```python
from build123d import *

# Parameters (mm, degrees)
CROQUIS1_R              = 8.85
SALIENTE_EXTRUIR1_DEPTH = 6.45
CROQUIS2_R              = 6
SALIENTE_EXTRUIR2_DEPTH = 12.9
CROQUIS3_R              = 8.85
SALIENTE_EXTRUIR3_DEPTH = 1.4
CROQUIS4_R              = 4
CORTAR_EXTRUIR1_DEPTH   = 25.232364722
CROQUIS6_W              = 1.65
CROQUIS6_H              = 8.851
MATRIZC1_COUNT          = 2
MATRIZC1_ANGLE          = 90


with BuildPart() as part:
    # Croquis1 → Saliente-Extruir1 (new body)
    with BuildSketch(Plane(origin=(0, 0, 0), x_dir=(1, 0, 0), z_dir=(0, 1, 0))):
        with Locations(Location((0, 0, 0), (0, 0, 90))):
            Circle(CROQUIS1_R)
    extrude(amount=SALIENTE_EXTRUIR1_DEPTH)

    # Croquis2 → Saliente-Extruir2 (add)
    with BuildSketch(Plane(origin=(0, 6.45, 0), x_dir=(1, 0, 0), z_dir=(0, 1, 0))):
        with Locations(Location((0, 0, 0), (0, 0, 90))):
            Circle(CROQUIS2_R)
    extrude(amount=SALIENTE_EXTRUIR2_DEPTH)

    # Croquis3 → Saliente-Extruir3 (add)
    with BuildSketch(Plane(origin=(0, 19.35, 0), x_dir=(1, 0, 0), z_dir=(0, 1, 0))):
        with Locations(Location((0, 0, 0), (0, 0, 90))):
            Circle(CROQUIS3_R)
    extrude(amount=SALIENTE_EXTRUIR3_DEPTH)

    # Croquis4 → Cortar-Extruir1 (cut, through all)
    with BuildSketch(Plane(origin=(0, 20.75, 0), x_dir=(1, 0, 0), z_dir=(0, 1, 0))):
        with Locations(Location((0, 0, 0), (0, 0, 270))):
            Circle(CROQUIS4_R)
    extrude(amount=-CORTAR_EXTRUIR1_DEPTH, mode=Mode.SUBTRACT)

    # Croquis6 → Taladro roscado M41 (falta definir posicio) (revolve, cut)
    with BuildSketch(Plane(origin=(0, 3.225, 0), x_dir=(0, 1, 0), z_dir=(1, 0, 0))):
        with Locations((0.825, 4.4255)):
            Rectangle(CROQUIS6_W, CROQUIS6_H)
    taladro_roscado_m41_falta_definir_posic = revolve(axis=Axis((0, 3.225, -6.35), (0, 0, 1)), mode=Mode.SUBTRACT)

    # MatrizC1: Taladro roscado M41 (falta definir posicio) ×2 about axis
    matrizc1_axis = Axis((0, 6.45, 0), (0, -1, 0))
    for i in range(1, MATRIZC1_COUNT):
        add(taladro_roscado_m41_falta_definir_posic.rotate(matrizc1_axis, i * MATRIZC1_ANGLE / (MATRIZC1_COUNT - 1)), mode=Mode.SUBTRACT)


solid = part.part
```
Could you check a few things on this model? Use its own coordinates, in mm. A direction names the side the tool comes from. Coordinates: 2 decimals unless noted, no trailing zeros. Write each loop counter-clockwise with the first axis right and the second up, starting at its lowest first coordinate (ties: lowest second). Pieces come first, ordered by that corner, then holes. Notation, with made-up numbers: (49.25, -2) -> (78.25, -2) arc R23 ccw to (78.25, 28) -> close; hole circle Ø5 at (-26, 14). An arc over 180 degrees is marked (long way). Return JSON: item names as keys, results as strings.
(1) We'd pull the mould along Y, two halves only. Please class faces 4 (the cylindrical face through (-2.66, 20.04, -8.44)), 5 (the flat face through (2, 6.45, -6)), 6 (the cylindrical face through (-6.29, 4.75, 0.63)), 7 (the flat face through (2, 20.75, -4)): +Y half, -Y half, draft (parallel to the pull), parting line (faces both ways), or undercut.
Numbers:
{"face 4": "draft", "face 5": "undercut", "face 6": "undercut", "face 7": "+Y half"}
(2) Which directions (+Z, -Z, +X, -X, +Y, -Y) give clear straight access to the entire face, cutting with the end or side of a thin tool? Please do faces 1 (the flat face through (2, 19.35, -6)), 2 (the cylindrical face through (0.63, 4.75, 6.28)), 3 (the cylindrical face through (3.39, 3.18, -8.175)).
Numbers:
{"face 1": "none", "face 2": "+Z", "face 3": "+Y, -Y"}
(3) Imagine slicing it at A-A, the plane x = 0. Please give me the cut outline in (y, z) (3 decimals), then the cut area to 3 significant figures.
Numbers:
{"outline": "(0, -8.85) -> (6.45, -8.85) -> (6.45, -6) -> (19.35, -6) -> (19.35, -8.85) -> (20.75, -8.85) -> (20.75, -4) -> (0, -4) -> close; (0, 4) -> (1.575, 4) -> (1.575, 8.85) -> (0, 8.85) -> close; (4.875, 4) -> (20.75, 4) -> (20.75, 8.85) -> (19.35, 8.85) -> (19.35, 6) -> (6.45, 6) -> (6.45, 8.85) -> (4.875, 8.85) -> close", "area": "112 mm2"}
(4) Imagine slicing it at C-C, the plane z = -3. Please give me the cut outline in (x, y), then the cut area to 3 significant figures.
Numbers:
{"outline": "(-8.33, 0) -> (-2.65, 0) -> (-2.65, 20.75) -> (-8.33, 20.75) -> (-8.33, 19.35) -> (-5.2, 19.35) -> (-5.2, 6.45) -> (-8.33, 6.45) -> close; (2.65, 0) -> (8.33, 0) -> (8.33, 6.45) -> (5.2, 6.45) -> (5.2, 19.35) -> (8.33, 19.35) -> (8.33, 20.75) -> (2.65, 20.75) -> close", "area": "155 mm2"}
(5) Imagine slicing it at B-B, the plane z = 0. Please give me the cut outline in (x, y) (3 decimals).
Numbers:
{"outline": "(-8.85, 0) -> (-4, 0) -> (-4, 1.575) -> (-8.85, 1.575) -> close; (-8.85, 4.875) -> (-4, 4.875) -> (-4, 20.75) -> (-8.85, 20.75) -> (-8.85, 19.35) -> (-6, 19.35) -> (-6, 6.45) -> (-8.85, 6.45) -> close; (4, 0) -> (8.85, 0) -> (8.85, 6.45) -> (6, 6.45) -> (6, 19.35) -> (8.85, 19.35) -> (8.85, 20.75) -> (4, 20.75) -> close"}
(6) I'm going to push flat-ended pins straight in: pin 1 (3 mm diameter, centred on y = 14, z = 2.5, fed in from -X); pin 2 (9 mm diameter, centred on x = 0, z = 0, fed in from +Y); pin 3 (4 mm diameter, centred on x = 6, y = 12.5, fed in from -Z); pin 4 (3 mm diameter, centred on x = 0, y = 3.225, fed in from +Z). Where does each tip first touch, or does it pass through?
Numbers:
{"pin 1": "stops at x = -5.92", "pin 2": "stops at y = 20.75", "pin 3": "stops at z = -4.47", "pin 4": "stops at z = -3.71"}
(7) Imagine slicing it at D-D, the plane x = -7.5. Please give me the cut outline in (y, z) (3 decimals).
Numbers:
{"outline": "(0, -4.698) -> (6.45, -4.698) -> (6.45, 4.698) -> (0, 4.698) -> close; (19.35, -4.698) -> (20.75, -4.698) -> (20.75, 4.698) -> (19.35, 4.698) -> close; hole circle Ø3.3 at (3.225, 0)"}
(8) I need wall thicknesses on L1, parallel to Y at x = 0, z = 7.2 (3 decimals); L2, parallel to Y at x = 2.75, z = -5.5; L3, parallel to X at y = 13, z = -1. Which ranges of each line are inside material? Lowest first, please.
Numbers:
{"L1": "y = 0 to 1.575, 4.875 to 6.45, 19.35 to 20.75", "L2": "y = 0 to 6.45, 19.35 to 20.75", "L3": "x = -5.92 to -3.87, 3.87 to 5.92"}
